```python
from build123d import *

# Parameters (mm, degrees)
SKETCH1_W           = 38.1
SKETCH1_H           = 12.7
BOSS_EXTRUDE1_DEPTH = 12.7
SKETCH2_R           = 5.1181
SKETCH2_R_2         = 1.8288
CUT_EXTRUDE1_DEPTH  = 12.7
SKETCH3_R           = 1.3335
CUT_EXTRUDE2_DEPTH  = 12.7


with BuildPart() as part:
    # Sketch1 → Boss-Extrude1 (new body)
    with BuildSketch(Plane(origin=(0, 0, 0), x_dir=(1, 0, 0), z_dir=(0, 1, 0))):
        Rectangle(SKETCH1_W, SKETCH1_H)
    extrude(amount=BOSS_EXTRUDE1_DEPTH)

    # Sketch2 → Cut-Extrude1 (cut)
    with BuildSketch(Plane(origin=(0, 12.7, 0), x_dir=(1, 0, 0), z_dir=(0, 1, 0))):
        with Locations(Location((0, 0, 0), (0, 0, 270))):
            Circle(SKETCH2_R)
        with Locations(Location((-12.7, 0, 0), (0, 0, 270))):
            Circle(SKETCH2_R_2)
        with Locations(Location((12.7, 0, 0), (0, 0, 270))):
            Circle(SKETCH2_R_2)
    extrude(amount=-CUT_EXTRUDE1_DEPTH, mode=Mode.SUBTRACT)

    # Sketch3 → Cut-Extrude2 (cut)
    with BuildSketch(Plane.XY.offset(6.35)):
        with Locations((-7.62, 6.35)):
            Circle(SKETCH3_R)
        with Locations((7.62, 6.35)):
            Circle(SKETCH3_R)
    extrude(amount=-CUT_EXTRUDE2_DEPTH, mode=Mode.SUBTRACT)


solid = part.part
```
Work out the finished part from the listing and answer in its coordinate system (mm). Give positions to 0.01 mm unless a question says otherwise; leave off trailing zeros. Loops run counter-clockwise (first coordinate to the right, second up) from the corner with the lowest first, then second, coordinate; pieces in that order, holes last. Notation, with made-up numbers: (86, -30.75) -> (141, -30.75) arc R24 ccw to (141, -17.75) -> close; hole circle Ø10 at (62.5, 53.5). An arc over 180 degrees is marked (long way). Put each result on its own line as item: value. Start each with the question number.
Item 1: Each of these flat-tipped pins is pushed along its axis until it touches: P1, Ø2, axis at x = -7.62, y = 6.35, coming from the -Z side; P2, Ø2, axis at x = -6, z = -0.5, coming from the -Y side. Where does it stop, or does it pass through?
Item 2: The mould has two halves that part along X. Classify faces 1 (the face through (14.513, 6.439, -0.238)), 2 (the face through (19.05, 6, 0)), 3 (the face through (-19.05, 6, 0)): released by +X, released by -X, zero draft, split by the parting line, or undercut.
Item 3: The part is cut by section A-A (y = 6.35). Give the vertices of the cut face in (x, z), then the cut area to 3 significant figures.
Item 4: The part is cut by section B-B (z = 0). Give the vertices of the cut face in (x, y), then the cut area to 3 significant figures.
Item 5: Find the intervals of material crossed by L1, parallel to X at y = 2.75, z = 0; L2, parallel to Y at x = 7.62, z = -2.5; L3, parallel to X at y = 5.5, z = 0, in increasing order. Write a range as [from, to].
Item 6: The part is cut by section C-C (x = 0). Give the vertices of the cut face in (y, z), then the cut area to 3 significant figures.
Item 7: The part is cut by section D-D (z = -4). Give the vertices of the cut face in (x, y).
Answers below:
1. P1: through
1. P2: y = 0
2. face 1: undercut
2. face 2: released by +X
2. face 3: released by -X
3. outline: (-19.05, -6.35) -> (-8.95, -6.35) -> (-8.95, 6.35) -> (-19.05, 6.35) -> close; (-6.29, -6.35) -> (6.29, -6.35) -> (6.29, 6.35) -> (-6.29, 6.35) -> close; (8.95, -6.35) -> (19.05, -6.35) -> (19.05, 6.35) -> (8.95, 6.35) -> close; hole circle Ø3.66 at (-12.7, 0); hole circle Ø10.24 at (0, 0); hole circle Ø3.66 at (12.7, 0)
3. area: 313 mm2
4. outline: (-19.05, 0) -> (-14.53, 0) -> (-14.53, 12.7) -> (-19.05, 12.7) -> close; (-10.87, 0) -> (-5.12, 0) -> (-5.12, 12.7) -> (-10.87, 12.7) -> close; (5.12, 0) -> (10.87, 0) -> (10.87, 12.7) -> (5.12, 12.7) -> close; (14.53, 0) -> (19.05, 0) -> (19.05, 12.7) -> (14.53, 12.7) -> close; hole circle Ø2.67 at (-7.62, 6.35); hole circle Ø2.67 at (7.62, 6.35)
4. area: 250 mm2
5. L1: [-19.05, -14.53], [-10.87, -5.12], [5.12, 10.87], [14.53, 19.05]
5. L2: [0, 5.02], [7.68, 12.7]
5. L3: [-19.05, -14.53], [-10.87, -8.65], [-6.59, -5.12], [5.12, 6.59], [8.65, 10.87], [14.53, 19.05]
6. outline: (0, -6.35) -> (12.7, -6.35) -> (12.7, -5.12) -> (0, -5.12) -> close; (0, 5.12) -> (12.7, 5.12) -> (12.7, 6.35) -> (0, 6.35) -> close
6. area: 31.3 mm2
7. outline: (-19.05, 0) -> (-3.19, 0) -> (-3.19, 12.7) -> (-19.05, 12.7) -> close; (3.19, 0) -> (19.05, 0) -> (19.05, 12.7) -> (3.19, 12.7) -> close; hole circle Ø2.67 at (-7.62, 6.35); hole circle Ø2.67 at (7.62, 6.35)
